The listing builds one solid part. Answer for the finished solid, in the listing's coordinates (mm). A direction names the side the tool comes from. Give positions to 0.01 mm unless a question says otherwise; leave off trailing zeros. Write each loop counter-clockwise with the first axis right and the second up, starting at its lowest first coordinate (ties: lowest second). Pieces come first, ordered by that corner, then holes. Notation, with made-up numbers: (25.5, 22) -> (34.5, 22) arc R7 ccw to (34.5, 29) -> close; hole circle Ø4 at (-18, 13.5). An arc over 180 degrees is marked (long way). Put each result on its own line as item: value. Start each with the question number.
1) Find the intervals of material crossed by line 1 along Y through (x, z) = (138, 1.45); line 2 along X through (y, z) = (85, 1.7); line 3 along Y through (x, z) = (94.5, 35.5), in increasing order. Write a range as from..to.
2) For a pull along X with two mould halves and no side action, classify faces 1 (the flat face through (134, 51, 4)), 2 (the flat face through (74, 13, 8)), 3 (the flat face through (43, 77, 36)) as released by +X, released by -X, zero draft, split by the parting line, or undercut.
3) A cutting plane is placed at C-C (y = 74). Write down the section's boundary in (x, z).
4) Flat-ended cylindrical pins translate along their axes: pin 1 Ø5 at (x, z) = (33.5, 31.5) entering from +Y; pin 2 Ø4 at (x, y) = (71, 88.5) entering from -Z; pin 3 Ø8 at (x, z) = (80.5, 14) entering from -Y; pin 4 Ø12 at (x, y) = (99, 15) entering from +Z. Find the tip coordinate at first contact, or state that the pin passes through.
5) A cutting plane is placed at A-A (x = 12). Write down the section's boundary in (y, z).
6) For faces 4 (the flat face through (105, 23, 21)), 5 (the flat face through (90, 20, 36)), 6 (the flat face through (108, 77, 36)), 7 (the flat face through (76, 87, 5)), determine the directions among +Z, -Z, +X, -X, +Y, -Y from which every point of the face is accessible in a straight line to the end or side of a thin tool.
7) A cutting plane is placed at D-D (x = 84.5). Write down the section's boundary in (y, z).
8) A cutting plane is placed at B-B (z = 19). Write down the section's boundary in (x, y).
from build123d import *

# Parameters (mm, degrees)
SKETCH1_W           = 150
SKETCH1_H           = 100
BOSS_EXTRUDE1_DEPTH = 4
SKETCH2_W           = 100
SKETCH2_H           = 100
BOSS_EXTRUDE2_DEPTH = 35
SKETCH3_W           = 100
SKETCH3_H           = 31
CUT_EXTRUDE1_DEPTH  = 20
SKETCH4_W           = 100
SKETCH4_H           = 35
CUT_EXTRUDE2_DEPTH  = 10
SKETCH5_W           = 30
SKETCH5_H           = 60
CUT_EXTRUDE3_DEPTH  = 95
SKETCH6_W           = 90
SKETCH6_H           = 5
CUT_EXTRUDE4_DEPTH  = 185.447824601
SKETCH7_W           = 75
SKETCH7_H           = 26
CUT_EXTRUDE5_DEPTH  = 5
SKETCH8_W           = 65
SKETCH8_H           = 15
CUT_EXTRUDE6_DEPTH  = 5
SKETCH9_W           = 15
SKETCH9_H           = 30
CUT_EXTRUDE7_DEPTH  = 5
SKETCH10_R          = 1.75
CUT_EXTRUDE8_DEPTH  = 5
FILLET1_R           = 1
FILLET2_R           = 1
FILLET3_R           = 1
FILLET4_R           = 1
FILLET5_R           = 1


with BuildPart() as part:
    # Sketch1 → Boss-Extrude1 (new body)
    with BuildSketch(Plane.XY):
        with Locations((75, 50)):
            Rectangle(SKETCH1_W, SKETCH1_H)
    extrude(amount=BOSS_EXTRUDE1_DEPTH)

    # Sketch2 → Boss-Extrude2 (add)
    with BuildSketch(Plane.XY.offset(4)):
        with Locations((75, 50)):
            Rectangle(SKETCH2_W, SKETCH2_H)
    extrude(amount=BOSS_EXTRUDE2_DEPTH)

    # Sketch3 → Cut-Extrude1 (cut)
    with BuildSketch(Plane(origin=(0, 0, 0), x_dir=(-1, 0, 0), z_dir=(0, -1, 0))):
        with Locations((-75, -23.5)):
            Rectangle(SKETCH3_W, SKETCH3_H)
    extrude(amount=-CUT_EXTRUDE1_DEPTH, mode=Mode.SUBTRACT)

    # Sketch4 → Cut-Extrude2 (cut)
    with BuildSketch(Plane(origin=(0, 100, 0), x_dir=(1, 0, 0), z_dir=(0, 1, 0))):
        with Locations((75, -21.5)):
            Rectangle(SKETCH4_W, SKETCH4_H)
    extrude(amount=-CUT_EXTRUDE2_DEPTH, mode=Mode.SUBTRACT)

    # Sketch5 → Cut-Extrude3 (cut)
    with BuildSketch(Plane(origin=(125, 0, 0), x_dir=(0, 0, -1), z_dir=(1, 0, 0))):
        with Locations((-19, 55)):
            Rectangle(SKETCH5_W, SKETCH5_H)
    extrude(amount=-CUT_EXTRUDE3_DEPTH, mode=Mode.SUBTRACT)

    # Sketch6 → Cut-Extrude4 (cut, through all)
    with BuildSketch(Plane(origin=(0, 0, 0), x_dir=(-1, 0, 0), z_dir=(0, -1, 0))):
        with Locations((-75, -2.5)):
            Rectangle(SKETCH6_W, SKETCH6_H)
    extrude(amount=-CUT_EXTRUDE4_DEPTH, mode=Mode.SUBTRACT)

    # Sketch7 → Cut-Extrude5 (cut)
    with BuildSketch(Plane(origin=(0, 20, 0), x_dir=(-1, 0, 0), z_dir=(0, -1, 0))):
        with Locations((-67.5, -21)):
            Rectangle(SKETCH7_W, SKETCH7_H)
    extrude(amount=-CUT_EXTRUDE5_DEPTH, mode=Mode.SUBTRACT)

    # Sketch8 → Cut-Extrude6 (cut)
    with BuildSketch(Plane.XY.offset(39)):
        with Locations((75.5, 77.5)):
            Rectangle(SKETCH8_W, SKETCH8_H)
    extrude(amount=-CUT_EXTRUDE6_DEPTH, mode=Mode.SUBTRACT)

    # Sketch9 → Cut-Extrude7 (cut)
    with BuildSketch(Plane.XY.offset(39)):
        with Locations((87.5, 40)):
            Rectangle(SKETCH9_W, SKETCH9_H)
    extrude(amount=-CUT_EXTRUDE7_DEPTH, mode=Mode.SUBTRACT)

    # Sketch10 → Cut-Extrude8 (cut)
    with BuildSketch(Plane.XY.offset(4)):
        with Locations((12, 85)):
            Circle(SKETCH10_R)
        with Locations((12, 19)):
            Circle(SKETCH10_R)
        with Locations((138, 85)):
            Circle(SKETCH10_R)
        with Locations((138, 19)):
            Circle(SKETCH10_R)
    extrude(amount=-CUT_EXTRUDE8_DEPTH, mode=Mode.SUBTRACT)

    # Fillet1
    fillet1_edges = [part.edges().sort_by_distance(p)[0] for p in [
        (10.25, 19, 4),
        (136.25, 85, 4),
        (136.25, 19, 4),
        (10.25, 85, 4),
    ]]
    fillet(fillet1_edges, radius=FILLET1_R)

    # Fillet2
    fillet2_edges = [part.edges().sort_by_distance(p)[0] for p in [
        (43, 77.5, 39),
        (75.5, 70, 39),
        (108, 77.5, 39),
        (75.5, 85, 39),
        (80, 40, 39),
        (87.5, 25, 39),
        (95, 40, 39),
        (87.5, 55, 39),
        (125, 55, 39),
        (75, 20, 39),
        (25, 55, 39),
        (75, 90, 39),
    ]]
    fillet(fillet2_edges, radius=FILLET2_R)

    # Fillet3
    # the kernel refuses this fillet: 1 mm, written as the material it takes off along each edge
    with BuildSketch(Plane(origin=(26, 21, 38), x_dir=(0, -1, 0), z_dir=(-1, 0, 0))) as fillet3_piece_1_section:
        Polygon((0, 0), (FILLET3_R, 0), (FILLET3_R, FILLET3_R), (0, FILLET3_R), align=None)
    fillet3_piece_1 = extrude(amount=FILLET3_R, mode=Mode.PRIVATE)
    fillet3_piece_1 = fillet3_piece_1 - Plane(origin=(26, 21, 38), x_dir=(0, 0.7071067811865475, -0.7071067811865475), z_dir=(-1, 0, 0)) * Sphere(FILLET3_R, mode=Mode.PRIVATE)
    add(fillet3_piece_1, mode=Mode.SUBTRACT)
    with BuildSketch(Plane(origin=(26, 89, 38), x_dir=(-1, 0, 0), z_dir=(0, 1, 0))) as fillet3_piece_2_section:
        Polygon((0, 0), (FILLET3_R, 0), (FILLET3_R, FILLET3_R), (0, FILLET3_R), align=None)
    fillet3_piece_2 = extrude(amount=FILLET3_R, mode=Mode.PRIVATE)
    fillet3_piece_2 = fillet3_piece_2 - Plane(origin=(26, 89, 38), x_dir=(0.7071067811865475, 0, -0.7071067811865475), z_dir=(0, 1, 0)) * Sphere(FILLET3_R, mode=Mode.PRIVATE)
    add(fillet3_piece_2, mode=Mode.SUBTRACT)
    with BuildSketch(Plane(origin=(124, 21, 38), x_dir=(0, -1, 0), z_dir=(1, 0, 0))) as fillet3_piece_3_section:
        Polygon((0, 0), (FILLET3_R, 0), (FILLET3_R, -FILLET3_R), (0, -FILLET3_R), align=None)
    fillet3_piece_3 = extrude(amount=FILLET3_R, mode=Mode.PRIVATE)
    fillet3_piece_3 = fillet3_piece_3 - Plane(origin=(124, 21, 38), x_dir=(0, 0.7071067811865475, -0.7071067811865475), z_dir=(1, 0, 0)) * Sphere(FILLET3_R, mode=Mode.PRIVATE)
    add(fillet3_piece_3, mode=Mode.SUBTRACT)
    with BuildSketch(Plane(origin=(124, 89, 38), x_dir=(1, 0, 0), z_dir=(0, 1, 0))) as fillet3_piece_4_section:
        Polygon((0, 0), (FILLET3_R, 0), (FILLET3_R, -FILLET3_R), (0, -FILLET3_R), align=None)
    fillet3_piece_4 = extrude(amount=FILLET3_R, mode=Mode.PRIVATE)
    fillet3_piece_4 = fillet3_piece_4 - Plane(origin=(124, 89, 38), x_dir=(-0.7071067811865475, 0, -0.7071067811865475), z_dir=(0, 1, 0)) * Sphere(FILLET3_R, mode=Mode.PRIVATE)
    add(fillet3_piece_4, mode=Mode.SUBTRACT)
    with BuildSketch(Plane(origin=(125, 90, 38), x_dir=(-1, 0, 0), z_dir=(0, 0, -1)), Plane(origin=(25, 90, 4), x_dir=(1, 0, 0), z_dir=(0, 0, 1))) as fillet3_piece_5:
        with BuildLine():
            CenterArc((FILLET3_R, -FILLET3_R), FILLET3_R, 90, 90)
            Line((0, -FILLET3_R), (0, 0))
            Line((0, 0), (FILLET3_R, 0))
        make_face()
    extrude(amount=34, mode=Mode.SUBTRACT)
    with BuildSketch(Plane(origin=(25, 20, 8), x_dir=(0, 1, 0), z_dir=(0, 0, 1)), Plane(origin=(125, 20, 38), x_dir=(0, 1, 0), z_dir=(0, 0, -1))) as fillet3_piece_6:
        with BuildLine():
            CenterArc((FILLET3_R, -FILLET3_R), FILLET3_R, 90, 90)
            Line((0, -FILLET3_R), (0, 0))
            Line((0, 0), (FILLET3_R, 0))
        make_face()
    extrude(amount=30, mode=Mode.SUBTRACT)
    with BuildSketch(Plane(origin=(25, -2.5, 8), x_dir=(0, 0, -1), z_dir=(0, 1, 0))) as fillet3_piece_7:
        with BuildLine():
            CenterArc((FILLET3_R, -FILLET3_R), FILLET3_R, 90, 90)
            Line((0, -FILLET3_R), (0, 0))
            Line((0, 0), (FILLET3_R, 0))
        make_face()
    extrude(amount=22.5, mode=Mode.SUBTRACT)
    with BuildSketch(Plane(origin=(125, -2.5, 8), x_dir=(0, 0, -1), z_dir=(0, 1, 0))) as fillet3_piece_8:
        with BuildLine():
            CenterArc((FILLET3_R, FILLET3_R), FILLET3_R, 180, 90)
            Line((0, FILLET3_R), (0, 0))
            Line((0, 0), (FILLET3_R, 0))
        make_face()
    extrude(amount=22.5, mode=Mode.SUBTRACT)
    with BuildSketch(Plane(origin=(127.5, 0, 8), x_dir=(0, 1, 0), z_dir=(-1, 0, 0))) as fillet3_piece_9:
        with BuildLine():
            CenterArc((FILLET3_R, FILLET3_R), FILLET3_R, 180, 90)
            Line((0, FILLET3_R), (0, 0))
            Line((0, 0), (FILLET3_R, 0))
        make_face()
    extrude(amount=105, mode=Mode.SUBTRACT)
    with BuildSketch(Plane(origin=(25, 20, 5.5), x_dir=(0, 1, 0), z_dir=(0, 0, 1))) as fillet3_piece_10a_section:
        with BuildLine():
            CenterArc((FILLET3_R, -FILLET3_R), FILLET3_R, 90, 90)
            Line((0, -FILLET3_R), (0, 0))
            Line((0, 0), (FILLET3_R, 0))
        make_face()
    fillet3_piece_10a = extrude(amount=32.5, mode=Mode.PRIVATE)
    fillet3_piece_10a = split(fillet3_piece_10a, bisect_by=Plane(origin=(25.226395114, 20.226395114, 8), z_dir=(0, 0, -1)), keep=Keep.TOP, mode=Mode.PRIVATE)
    with BuildSketch(Plane(origin=(25, -2.5, 8), x_dir=(0, 0, -1), z_dir=(0, 1, 0))) as fillet3_piece_10b_section:
        with BuildLine():
            CenterArc((FILLET3_R, -FILLET3_R), FILLET3_R, 90, 90)
            Line((0, -FILLET3_R), (0, 0))
            Line((0, 0), (FILLET3_R, 0))
        make_face()
    fillet3_piece_10b = extrude(amount=25, mode=Mode.PRIVATE)
    fillet3_piece_10b = split(fillet3_piece_10b, bisect_by=Plane(origin=(25.226395114, 20, 7.773604886), z_dir=(0, 1, 0)), keep=Keep.TOP, mode=Mode.PRIVATE)
    fillet3_piece_10 = fillet3_piece_10a & fillet3_piece_10b
    add(fillet3_piece_10, mode=Mode.SUBTRACT)
    with BuildSketch(Plane(origin=(125, 20, 38), x_dir=(0, 1, 0), z_dir=(0, 0, -1))) as fillet3_piece_11a_section:
        with BuildLine():
            CenterArc((FILLET3_R, -FILLET3_R), FILLET3_R, 90, 90)
            Line((0, -FILLET3_R), (0, 0))
            Line((0, 0), (FILLET3_R, 0))
        make_face()
    fillet3_piece_11a = extrude(amount=32.5, mode=Mode.PRIVATE)
    fillet3_piece_11a = split(fillet3_piece_11a, bisect_by=Plane(origin=(124.773604886, 20.226395114, 8), z_dir=(0, 0, -1)), keep=Keep.TOP, mode=Mode.PRIVATE)
    with BuildSketch(Plane(origin=(125, -2.5, 8), x_dir=(0, 0, -1), z_dir=(0, 1, 0))) as fillet3_piece_11b_section:
        with BuildLine():
            CenterArc((FILLET3_R, FILLET3_R), FILLET3_R, 180, 90)
            Line((0, FILLET3_R), (0, 0))
            Line((0, 0), (FILLET3_R, 0))
        make_face()
    fillet3_piece_11b = extrude(amount=25, mode=Mode.PRIVATE)
    fillet3_piece_11b = split(fillet3_piece_11b, bisect_by=Plane(origin=(124.773604886, 20, 7.773604886), z_dir=(0, 1, 0)), keep=Keep.TOP, mode=Mode.PRIVATE)
    fillet3_piece_11 = fillet3_piece_11a & fillet3_piece_11b
    add(fillet3_piece_11, mode=Mode.SUBTRACT)

    # Fillet4
    fillet4_edges = [part.edges().sort_by_distance(p)[0] for p in [
        (12.5, 0, 4),
        (137.5, 0, 4),
        (0, 50, 4),
        (15, 100, 4),
        (135, 100, 4),
        (30, 95, 4),
        (120, 95, 4),
        (150, 50, 4),
    ]]
    fillet(fillet4_edges, radius=FILLET4_R)

    # Fillet5
    fillet5_edges = [part.edges().sort_by_distance(p)[0] for p in [
        (30, 20, 21),
        (105, 20, 21),
        (67.5, 20, 34),
    ]]
    fillet(fillet5_edges, radius=FILLET5_R)


solid = part.part
Reply:
1. line 1: y = 0..17.25, 20.75..83.25, 86.75..100
1. line 2: x = 0..10.25, 13.75..30, 120..136.25, 139.75..150
1. line 3: y = 20..25, 55..70, 85..90
2. face 1: zero draft
2. face 2: undercut
2. face 3: undercut
3. outline: (0, 0) -> (30, 0) -> (30, 34) -> (43, 34) -> (43, 38) arc R1 ccw to (42, 39) -> (26, 39) arc R1 ccw to (25, 38) -> (25, 4) -> (1, 4) arc R1 ccw to (0, 3) -> close; (108, 34) -> (125, 34) -> (125, 38) arc R1 ccw to (124, 39) -> (109, 39) arc R1 ccw to (108, 38) -> close; (120, 0) -> (150, 0) -> (150, 3) arc R1 ccw to (149, 4) -> (120, 4) -> close
4. pin 1: stops at y = 90
4. pin 2: stops at z = 5
4. pin 3: stops at y = 85
4. pin 4: stops at z = 39
5. outline: (0, 0) -> (17.25, 0) -> (17.25, 3) arc R1 ccw to (16.25, 4) -> (1, 4) arc R1 ccw to (0, 3) -> close; (20.75, 0) -> (83.25, 0) -> (83.25, 3) arc R1 ccw to (82.25, 4) -> (21.75, 4) arc R1 ccw to (20.75, 3) -> close; (86.75, 0) -> (100, 0) -> (100, 3) arc R1 ccw to (99, 4) -> (87.75, 4) arc R1 ccw to (86.75, 3) -> close
6. face 4: -Y
6. face 5: +Z, +X, -X, -Y
6. face 6: +Z, -Z
6. face 7: -Z, +Y, -Y
7. outline: (0, 5) -> (25, 5) -> (25, 8) -> (1, 8) arc R1 ccw to (0, 7) -> close; (20, 35) arc R1 ccw to (21, 34) -> (25, 34) -> (25, 38) arc R1 ccw to (24, 39) -> (21, 39) arc R1 ccw to (20, 38) -> close; (55, 34) -> (70, 34) -> (70, 38) arc R1 ccw to (69, 39) -> (56, 39) arc R1 ccw to (55, 38) -> close; (85, 5) -> (90, 5) -> (90, 38) arc R1 ccw to (89, 39) -> (86, 39) arc R1 ccw to (85, 38) -> close
8. outline: (25, 21) arc R1 ccw to (26, 20) -> (29, 20) arc R1 ccw to (30, 21) -> (30, 85) -> (125, 85) -> (125, 89) arc R1 ccw to (124, 90) -> (26, 90) arc R1 ccw to (25, 89) -> close; (105, 21) arc R1 ccw to (106, 20) -> (124, 20) arc R1 ccw to (125, 21) -> (125, 25) -> (105, 25) -> close
